Source: CAD feature listing. Evaluate the final solid. Frame: model axes, mm. A direction names the side the tool comes from. Give positions to 0.01 mm unless a question says otherwise; leave off trailing zeros. Order: outer loops, then holes, each group sorted by start corner. A loop starts at its lowest first (then second) coordinate and runs counter-clockwise, first axis right, second up. Notation, with made-up numbers: (62.25, -27.75) - (91.25, -27.75) arc R15 ccw to (91.25, -7.75) - close; hole circle Ø11 at (-30, 74). An arc over 180 degrees is marked (long way). Use CSV: the item, a comma, the result in double quotes.
```python
from build123d import *

# Parameters (mm, degrees)
SKETCH1_W                       = 101.6
SKETCH1_H                       = 63.5
BOSS_EXTRUDE1_DEPTH             = 9.525
F_8_32_TAPPED_HOLE1_D           = 3.4544
F_8_32_TAPPED_HOLE1_DEPTH       = 19.05
F_8_32_TAPPED_HOLE1_CSINK_D     = 4.1656
F_8_32_TAPPED_HOLE1_CSINK_ANGLE = 90
F_8_32_TAPPED_HOLE1_TIP         = 1.037806461
F_8_CLEARANCE_HOLE2_D           = 4.4958
F_8_CLEARANCE_HOLE2_DEPTH       = 25.4
F_8_CLEARANCE_HOLE2_TIP         = 1.350674586
F_6_32_TAPPED_HOLE1_D           = 2.7051
F_4_CLEARANCE_HOLE1_D           = 3.2639
F_4_CLEARANCE_HOLE1_DEPTH       = 9.525


with BuildPart() as part:
    # Sketch1 → Boss-Extrude1 (new body)
    with BuildSketch(Plane.XY):
        with Locations((-50.8, 31.75)):
            Rectangle(SKETCH1_W, SKETCH1_H)
    extrude(amount=BOSS_EXTRUDE1_DEPTH)

    # #8-32 Tapped Hole1
    with Locations(Plane(origin=(0, 63.5, 0), x_dir=(1, 0, 0), z_dir=(0, 1, 0))):
        with Locations((-44.45, -4.7625), (-57.15, -4.7625)):
            CounterSinkHole(F_8_32_TAPPED_HOLE1_D / 2, F_8_32_TAPPED_HOLE1_CSINK_D / 2, depth=F_8_32_TAPPED_HOLE1_DEPTH, counter_sink_angle=F_8_32_TAPPED_HOLE1_CSINK_ANGLE)
            with Locations((0, 0, -(F_8_32_TAPPED_HOLE1_DEPTH + F_8_32_TAPPED_HOLE1_TIP / 2))):  # 118° drill point
                Cone(0, F_8_32_TAPPED_HOLE1_D / 2, F_8_32_TAPPED_HOLE1_TIP, mode=Mode.SUBTRACT)

    # #8 Clearance Hole2
    with Locations(Plane.XY.offset(9.525)):
        with Locations((-44.45, 43.412193539), (-57.15, 43.412193539)):
            Hole(F_8_CLEARANCE_HOLE2_D / 2, depth=F_8_CLEARANCE_HOLE2_DEPTH)
            with Locations((0, 0, -(F_8_CLEARANCE_HOLE2_DEPTH + F_8_CLEARANCE_HOLE2_TIP / 2))):  # 118° drill point
                Cone(0, F_8_CLEARANCE_HOLE2_D / 2, F_8_CLEARANCE_HOLE2_TIP, mode=Mode.SUBTRACT)

    # #6-32 Tapped Hole1 (through all)
    with Locations(Plane.XY.offset(9.525)):
        with Locations((-95.25, 6.35), (-95.25, 57.15), (-6.35, 6.35), (-6.35, 57.15)):
            Hole(F_6_32_TAPPED_HOLE1_D / 2)

    # #4 Clearance Hole1
    with Locations(Plane.XY.offset(9.525)):
        with Locations((-82.55, 12.7), (-19.05, 12.7)):
            Hole(F_4_CLEARANCE_HOLE1_D / 2, depth=F_4_CLEARANCE_HOLE1_DEPTH)


solid = part.part
```
Item 1: First-contact query: pin 1 (4.5 mm diameter, centred on x = -6.35, y = 57.15, fed in from -Z); pin 2 (3 mm diameter, centred on x = -44.45, z = 4.76, fed in from +Y); pin 3 (1 mm diameter, centred on x = -56.5, z = 5.5, fed in from +Y). Flat tips, straight axial feed; report the tip coordinate or a pass-through.
Filled in:
pin 1,"stops at z = 0"
pin 2,"stops at y = 41.74"
pin 3,"stops at y = 41.48"
Item 2: Section D-D on y = 57.15. Count the separate pieces of the cut face and the enclosed holes in it, then the cut area to 3 significant figures.
Filled in:
separate pieces,"3"
enclosed holes,"2"
area,"897 mm2"
Item 3: Section A-A on x = -6.35. Return the cut outline in (y, z) (3 decimals), then the cut area to 3 significant figures.
Filled in:
outline,"(0, 0) - (4.997, 0) - (4.997, 9.525) - (0, 9.525) - close; (7.703, 0) - (55.797, 0) - (55.797, 9.525) - (7.703, 9.525) - close; (58.503, 0) - (63.5, 0) - (63.5, 9.525) - (58.503, 9.525) - close"
area,"553 mm2"
Item 4: Set-up query: faces 5 (the cylindrical face through (-43.177, 53.87, 3.595)), 6 (the cylindrical face through (-56.66, 41.22, 4.7)). Return all of +Z, -Z, +X, -X, +Y, -Y with unobstructed straight access to the full face (end or side cutting, diameter ignored); none if empty.
Filled in:
face 5,"+Y"
face 6,"+Z, -Z"
Item 5: Material intervals for line 1 (Y direction, x = -6.35, z = 2.5); line 2 (Y direction, x = -19.05, z = 3); line 3 (Y direction, x = -57.15, z = 4.75), sorted ascending. Write a range as from..to.
Filled in:
line 1,"y = 0..5, 7.7..55.8, 58.5..63.5"
line 2,"y = 0..11.07, 14.33..63.5"
line 3,"y = 0..41.16"
Item 6: Mould query, pull axis Y, two halves, no side actions, for faces 1 (the flat face through (-52, 0, 5)), 2 (the cylindrical face through (-20.607, 13.19, 4.696)), 3 (the cylindrical face through (-43.96, 41.22, 4.7)), 4 (the cylindrical face through (-55.424, 53.87, 4.687)). Classes: released by +Y, released by -Y, zero draft, split by the parting line, or undercut.
Filled in:
face 1,"released by -Y"
face 2,"undercut"
face 3,"undercut"
face 4,"zero draft"
Item 7: Section B-B on x = -19.05. Return the cut outline in (y, z) (3 decimals), then the cut area to 3 significant figures.
Filled in:
outline,"(0, 0) - (11.068, 0) - (11.068, 9.525) - (0, 9.525) - close; (14.332, 0) - (63.5, 0) - (63.5, 9.525) - (14.332, 9.525) - close"
area,"574 mm2"
Item 8: Section C-C on y = 6.35. Return the cut outline in (x, z) (3 decimals), then the cut area to 3 significant figures.
Filled in:
outline,"(-101.6, 0) - (-96.603, 0) - (-96.603, 9.525) - (-101.6, 9.525) - close; (-93.897, 0) - (-7.703, 0) - (-7.703, 9.525) - (-93.897, 9.525) - close; (-4.997, 0) - (0, 0) - (0, 9.525) - (-4.997, 9.525) - close"
area,"916 mm2"
